from build123d import *

# Parameters (mm, degrees)
F0_W     = 50
F0_H     = 57
F1_DEPTH = 50
F2_R     = 5
F3_DEPTH = 50.001
F4_R     = 5
F5_DEPTH = 50.001
F4_R_2   = 11
F6_DEPTH = 8
F7_START = -43
F7_DEPTH = 7
F2_R_2   = 12.1936245424
F8_DEPTH = 10


with BuildPart() as f1:
    # F0 (on Top) → F1 (new body)
    with BuildSketch(Plane.XY):
        with Locations((25, 28.5)):
            Rectangle(F0_W, F0_H)
    extrude(amount=F1_DEPTH)

    # F2 (on face) → F3 (cut, through all)
    with BuildSketch(Plane.XY.offset(50)):
        with Locations((25, 15)):
            Circle(F2_R)
    extrude(amount=-F3_DEPTH, mode=Mode.SUBTRACT)

    # F4 (on face) → F5 (cut, through all)
    with BuildSketch(Plane(origin=(0, 0, 0), x_dir=(0, -1, 0), z_dir=(-1, 0, 0))):
        with Locations((-41, 30)):
            Circle(F4_R)
    extrude(amount=-F5_DEPTH, mode=Mode.SUBTRACT)

    # F4 (on face) → F6 (cut)
    with BuildSketch(Plane(origin=(0, 0, 0), x_dir=(0, -1, 0), z_dir=(-1, 0, 0))):
        with Locations((-41, 30)):
            Circle(F4_R_2)
        with Locations((-41, 30)):
            Circle(F4_R, mode=Mode.SUBTRACT)
    extrude(amount=-F6_DEPTH, mode=Mode.SUBTRACT)

    # F4 (on face) → F7 (cut)
    with BuildSketch(Plane(origin=(0, 0, 0), x_dir=(0, -1, 0), z_dir=(-1, 0, 0)).offset(F7_START)):
        with Locations((-41, 30)):
            Circle(F4_R_2)
        with Locations((-41, 30)):
            Circle(F4_R, mode=Mode.SUBTRACT)
    extrude(amount=-F7_DEPTH, mode=Mode.SUBTRACT)

    # F2 (on face) → F8 (cut)
    with BuildSketch(Plane.XY.offset(50)):
        with Locations((25, 15)):
            Circle(F2_R_2)
        with Locations((25, 15)):
            Circle(F2_R, mode=Mode.SUBTRACT)
    extrude(amount=-F8_DEPTH, mode=Mode.SUBTRACT)


solid = f1.part
Could you check a few things on this model? Use its own coordinates, in mm. A direction names the side the tool comes from. Coordinates: 2 decimals unless noted, no trailing zeros. Order: outer loops, then holes, each group sorted by start corner. A loop starts at its lowest first (then second) coordinate and runs counter-clockwise, first axis right, second up. Notation, with made-up numbers: (-3.75, 89.5) - (50.25, 89.5) arc R23 ccw to (50.25, 99.5) - close; hole circle Ø5 at (77.25, 2.25). An arc over 180 degrees is marked (long way). Answer in a Markdown table with one row per item. Add a question column.
(1) If we mould it in two halves opening along Z, with no side actions, what happens to faces 1 (the face through (21, 12, 20)), 2 (the face through (24.8, 9.8, 40)), 3 (the face through (25, 29, 0)), 4 (the face through (25, 46, 30))? For each: released by +Z, released by -Z, zero draft, split by the parting line, or undercut.
(2) If we section it at D-D, the plane z = 23: Please give me the cut outline in (x, y).
(3) If we section it at A-A, the plane z = 30: Please give me the cut outline in (x, y), then the cut area to 3 significant figures.
(4) If we section it at B-B, the plane y = 41: Please give me the cut outline in (x, z).
(5) On a 3-axis mill with a long thin cutter (end or side, diameter ignored), from which of +Z, -Z, +X, -X, +Y, -Y can I reach the whole of each face in a straight line? I mean faces 5 (the face through (25, 57, 25)), 6 (the face through (8, 39, 25)), 7 (the face through (43, 39, 25)), 8 (the face through (0, 28, 25)), 9 (the face through (23.41, 27.09, 45.07)). Say none if no direction works.
(6) Will these pins go through, and if not, where does the flat tip stop? pin 1 (6.5 mm diameter, centred on y = 38.5, z = 35, fed in from -X); pin 2 (1 mm diameter, centred on x = 22.5, y = 15, fed in from +Z); pin 3 (7.5 mm diameter, centred on x = 24.5, y = 13.5, fed in from +Z).
(7) If we section it at C-C, the plane x = 22: Please give me the cut outline in (y, z).
(8) I need wall thicknesses on L1, parallel to Z at x = 6, y = 41; L2, parallel to Z at x = 19, y = 41; L3, parallel to Z at x = 16.5, y = 13. Which ranges of each line are inside material? Lowest first, please.
Results are:
| question | item | result |
|---|---|---|
| 1 | face 1 | zero draft |
| 1 | face 2 | released by +Z |
| 1 | face 3 | released by -Z |
| 1 | face 4 | undercut |
| 2 | outline | (0, 0) - (50, 0) - (50, 32.51) - (43, 32.51) - (43, 49.49) - (50, 49.49) - (50, 57) - (0, 57) - (0, 49.49) - (8, 49.49) - (8, 32.51) - (0, 32.51) - close; hole circle Ø10 at (25, 15) |
| 3 | outline | (0, 0) - (50, 0) - (50, 30) - (43, 30) - (43, 36) - (8, 36) - (8, 30) - (0, 30) - close; (0, 52) - (8, 52) - (8, 46) - (43, 46) - (43, 52) - (50, 52) - (50, 57) - (0, 57) - close; hole circle Ø10 at (25, 15) |
| 3 | area | 2,090 mm2 |
| 4 | outline | (0, 0) - (50, 0) - (50, 19) - (43, 19) - (43, 25) - (8, 25) - (8, 19) - (0, 19) - close; (0, 41) - (8, 41) - (8, 35) - (43, 35) - (43, 41) - (50, 41) - (50, 50) - (0, 50) - close |
| 5 | face 5 | +Z, -Z, +X, -X, +Y |
| 5 | face 6 | -X |
| 5 | face 7 | +X |
| 5 | face 8 | +Z, -Z, -X, +Y, -Y |
| 5 | face 9 | +Z |
| 6 | pin 1 | stops at x = 8 |
| 6 | pin 2 | passes through |
| 6 | pin 3 | stops at z = 40 |
| 7 | outline | (0, 0) - (11, 0) - (11, 40) - (3.18, 40) - (3.18, 50) - (0, 50) - close; (19, 0) - (57, 0) - (57, 50) - (26.82, 50) - (26.82, 40) - (19, 40) - close; hole circle Ø10 at (41, 30) |
| 8 | L1 | z = 0 to 19, 41 to 50 |
| 8 | L2 | z = 0 to 25, 35 to 50 |
| 8 | L3 | z = 0 to 40 |
